Part model, mm, in its own coordinate system. A direction names the side the tool comes from. Give positions to 0.01 mm unless a question says otherwise; leave off trailing zeros. Order: outer loops, then holes, each group sorted by start corner. A loop starts at its lowest first (then second) coordinate and runs counter-clockwise, first axis right, second up. Notation, with made-up numbers: M 46.5,-10.75 L 96.5,-10.75 A16 cw 96.5,8.25 Z; hole C 12,39.5 d9. An arc over 180 degrees is marked long. Return JSON: item names as keys, results as strings.
from build123d import *

# Parameters (mm, degrees)
F0_W     = 60
F0_H     = 28
F1_DEPTH = 50
F2_R     = 7
F3_DEPTH = 50
F4_R     = 7
F5_DEPTH = 50


with BuildPart() as f1:
    # F0 (on Right) → F1 (new body, symmetric)
    with BuildSketch(Plane.YZ):
        Polygon((-502.916585, 14), (-502.916585, 0), (497.083415, 0), (497.083415, 14), (437.083415, 14), (-442.916585, 14), align=None)
        with Locations((-472.916585, 28)):
            Rectangle(F0_W, F0_H)
        with Locations((467.083415, 28)):
            Rectangle(F0_W, F0_H)
    extrude(amount=F1_DEPTH, both=True)

    # F2 (on face) → F3 (cut, symmetric)
    with BuildSketch(Plane.XY.offset(42)):
        with Locations((-30, -472.916585)):
            Circle(F2_R)
        with BuildLine():
            ThreePointArc((37, -472.916585), (30, -465.916585), (23, -472.916585))
            ThreePointArc((23, -472.916585), (30, -479.916585), (37, -472.916585))
        make_face()
    extrude(amount=F3_DEPTH, both=True, mode=Mode.SUBTRACT)

    # F4 (on face) → F5 (cut, symmetric)
    with BuildSketch(Plane.XY.offset(42)):
        with Locations((-30, 467.083415)):
            Circle(F4_R)
        with BuildLine():
            ThreePointArc((37, 467.083415), (30, 474.083415), (23, 467.083415))
            ThreePointArc((23, 467.083415), (30, 460.083415), (37, 467.083415))
        make_face()
    extrude(amount=F5_DEPTH, both=True, mode=Mode.SUBTRACT)


solid = f1.part
Q1. Band-saw the part on B-B (x = -6). Give the cut face in (y, z), then the cut area to 3 significant figures.
Established:
{"outline": "M -502.92,0 L 497.08,0 L 497.08,42 L 437.08,42 L 437.08,14 L -442.92,14 L -442.92,42 L -502.92,42 Z", "area": "17,400 mm²"}
Q2. Band-saw the part on C-C (y = 301.5). Give the cut face in (x, z).
Established:
{"outline": "M -50,0 L 50,0 L 50,14 L -50,14 Z"}
Q3. Band-saw the part on A-A (z = 29). Give the cut face in (x, y).
Established:
{"outline": "M -50,-502.92 L 50,-502.92 L 50,-442.92 L -50,-442.92 Z; M -50,437.08 L 50,437.08 L 50,497.08 L -50,497.08 Z; hole C -30,-472.92 d14; hole C -30,467.08 d14; hole C 30,-472.92 d14; hole C 30,467.08 d14"}
Q4. Two-plate mould, pull along Y, no slides. Class faces 3 (the flat face through (1, 437.083, 28)), 4 (the flat face through (1, -502.917, 21)), 5 (the flat face through (1, 467, 42)): +Y half, -Y half, draft (parallel to the pull), parting line (faces both ways), or undercut.
Established:
{"face 3": "undercut", "face 4": "-Y half", "face 5": "draft"}
Q5. 3-axis set-ups, long thin cutter, end or side, ignore diameter. For faces 1 (the flat face through (1, 497.083, 21)), 2 (the flat face through (1, -442.917, 28)): which of +Z, -Z, +X, -X, +Y, -Y reach the whole face in a straight line?
Established:
{"face 1": "+Z, -Z, +X, -X, +Y", "face 2": "+Z, +X, -X"}
Q6. Probe line 1 along Y through (x, z) = (-30, 9.5); line 2 along Y through (x, z) = (30, 22); line 3 along Y through (x, z) = (5.5, 30.5). List the from-to ranges inside material, lowest first.
Established:
{"line 1": "y = -502.92 to -479.92, -465.92 to 460.08, 474.08 to 497.08", "line 2": "y = -502.92 to -479.92, -465.92 to -442.92, 437.08 to 460.08, 474.08 to 497.08", "line 3": "y = -502.92 to -442.92, 437.08 to 497.08"}
Q7. Pin check, flat tip, straight feed: pin 1 (1.5 mm diameter, centred on x = 39.5, y = 373.5, fed in from +Z). Stop position of the tip, or through.
Established:
{"pin 1": "stops at z = 14"}
